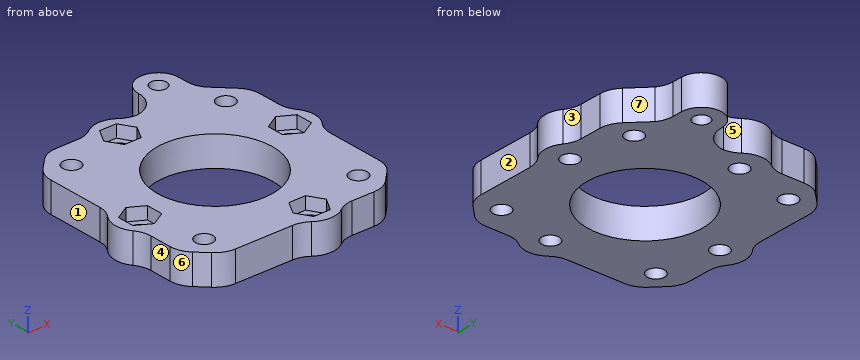
from build123d import *

# Parameters (mm, degrees)
SKETCH1_R           = 11.5
BOSS_EXTRUDE1_DEPTH = 6
SKETCH5_R           = 4.951700006
BOSS_EXTRUDE3_DEPTH = 6
SKETCH2_R           = 1.75
CUT_EXTRUDE1_DEPTH  = 34.075670817
SKETCH3_R           = 1.75
CUT_EXTRUDE2_DEPTH  = 34.075670817
CUT_EXTRUDE3_DEPTH  = 2.5
SKETCH6_R           = 1.6
BOSS_EXTRUDE4_DEPTH = 6
FILLET1_R           = 5


with BuildPart() as part:
    # Sketch1 → Boss-Extrude1 (new body)
    with BuildSketch(Plane.XY):
        Polygon((-21, 16), (-16, 21), (16, 21), (21, 16), (21, -16), (16, -21), (-16, -21), (-21, -16), align=None)
        Circle(SKETCH1_R, mode=Mode.SUBTRACT)
    extrude(amount=BOSS_EXTRUDE1_DEPTH)

    # Sketch5 → Boss-Extrude3 (add)
    with BuildSketch(Plane(origin=(0, 0, 0), x_dir=(-1, 0, 0), z_dir=(0, 0, -1))):
        with Locations((-18.048299994, 3.501266534)):
            Circle(SKETCH5_R)
        with Locations((3.501266534, 18.048299994)):
            Circle(SKETCH5_R)
        with Locations((18.048299994, -3.501266534)):
            Circle(SKETCH5_R)
        with Locations((-3.501266534, -18.048299994)):
            Circle(SKETCH5_R)
    extrude(amount=-BOSS_EXTRUDE3_DEPTH)

    # Sketch2 → Cut-Extrude1 (cut, through all)
    with BuildSketch(Plane.XY.offset(6)):
        with Locations((-15.5, 15.5)):
            Circle(SKETCH2_R)
        with Locations((15.5, 15.5)):
            Circle(SKETCH2_R)
        with Locations((15.5, -15.5)):
            Circle(SKETCH2_R)
        with Locations((-15.5, -15.5)):
            Circle(SKETCH2_R)
    extrude(amount=-CUT_EXTRUDE1_DEPTH, mode=Mode.SUBTRACT)

    # Sketch3 → Cut-Extrude2 (cut, through all)
    with BuildSketch(Plane.XY.offset(6)):
        with Locations((-3.501266534, 18.048299994)):
            Circle(SKETCH3_R)
        with Locations((18.048299994, 3.501266534)):
            Circle(SKETCH3_R)
        with Locations((3.501266534, -18.048299994)):
            Circle(SKETCH3_R)
        with Locations((-18.048299994, -3.501266534)):
            Circle(SKETCH3_R)
    extrude(amount=-CUT_EXTRUDE2_DEPTH, mode=Mode.SUBTRACT)

    # Sketch4 → Cut-Extrude3 (cut)
    with BuildSketch(Plane.XY.offset(6)):
        Polygon((-0.152634973, 18.048299994), (-1.826950753, 20.948299994), (-5.175582315, 20.948299994), (-6.849898095, 18.048299994), (-5.175582315, 15.148299994), (-1.826950753, 15.148299994), align=None)
        Polygon((18.048299994, 6.849898095), (15.148299994, 5.175582315), (15.148299994, 1.826950753), (18.048299994, 0.152634973), (20.948299994, 1.826950753), (20.948299994, 5.175582315), align=None)
        Polygon((-18.048299994, -6.849898095), (-15.148299994, -5.175582315), (-15.148299994, -1.826950753), (-18.048299994, -0.152634973), (-20.948299994, -1.826950753), (-20.948299994, -5.175582315), align=None)
        Polygon((6.849898095, -18.048299994), (5.175582315, -15.148299994), (1.826950753, -15.148299994), (0.152634973, -18.048299994), (1.826950753, -20.948299994), (5.175582315, -20.948299994), align=None)
    extrude(amount=-CUT_EXTRUDE3_DEPTH, mode=Mode.SUBTRACT)

    # Sketch6 → Boss-Extrude4 (add)
    with BuildSketch(Plane(origin=(0, 0, 0), x_dir=(-1, 0, 0), z_dir=(0, 0, -1))):
        with BuildLine():
            Line((-15, 26), (-15, 21))
            Line((-15, 21), (-7, 21))
            Line((-7, 21), (-7, 26))
            ThreePointArc((-7, 26), (-11, 30), (-15, 26))
        make_face()
        with Locations((-11, 26)):
            Circle(SKETCH6_R, mode=Mode.SUBTRACT)
    extrude(amount=-BOSS_EXTRUDE4_DEPTH)

    # Fillet1
    # the kernel refuses this fillet: 5 mm, written as the material it adds along each edge
    with BuildSketch(Plane(origin=(15, 21, 0), x_dir=(1, 0, 0), z_dir=(0, 0, 1))) as fillet1_piece_1:
        with BuildLine():
            CenterArc((5, 3), FILLET1_R, 180, 36.869897646)
            Line((0, 3), (0, 0))
            Line((0, 0), (1, 0))
        make_face()
    extrude(amount=6)
    with BuildSketch(Plane(origin=(7, 21, 0), x_dir=(-1, 0, 0), z_dir=(0, 0, 1))) as fillet1_piece_2:
        with BuildLine():
            CenterArc((FILLET1_R, -FILLET1_R), FILLET1_R, 90, 90)
            Line((0, -FILLET1_R), (0, 0))
            Line((0, 0), (FILLET1_R, 0))
        make_face()
    extrude(amount=6)
    with BuildSketch(Plane(origin=(7.477043191, -21, 6), x_dir=(-0.7048105163679362, -0.7093956131927819, 0), z_dir=(0, 0, -1)), Plane(origin=(-21, -7.477043191, 6), x_dir=(-0.7093956131927642, 0.7048105163679541, 0), z_dir=(0, 0, -1))) as fillet1_piece_3:
        with BuildLine():
            CenterArc((2.13164688, -4.948591109), FILLET1_R, 98.223270181, 36.962491831)
            Line((-1.415331186, -1.424538527), (0, 0))
            ThreePointArc((0, 0), (0.708246162, -0.050912281), (1.416492325, 0))
        make_face()
    extrude(amount=6)
    with BuildSketch(Plane(origin=(-0.474510123, -21, 6), x_dir=(-1, 0, 0), z_dir=(0, 0, -1)), Plane(origin=(-21, 0.474510123, 6), x_dir=(0, 1, 0), z_dir=(0, 0, -1))) as fillet1_piece_4:
        with BuildLine():
            CenterArc((2.008101686, -5), FILLET1_R, 90, 36.962491831)
            ThreePointArc((-0.998358687, -1.004853441), (-0.463062395, -0.538310232), (0, 0))
            Line((0, 0), (2.008101686, 0))
        make_face()
    extrude(amount=6)
    with BuildSketch(Plane(origin=(-7.477043191, 21, 6), x_dir=(-1, 0, 0), z_dir=(0, 0, -1)), Plane(origin=(21, 7.477043191, 6), x_dir=(0, 1, 0), z_dir=(0, 0, -1))) as fillet1_piece_5:
        with BuildLine():
            CenterArc((2.008101686, 5), FILLET1_R, 233.037508169, 36.962491831)
            ThreePointArc((-0.998358687, 1.004853441), (-0.463062395, 0.538310232), (0, 0))
            Line((0, 0), (2.008101686, 0))
        make_face()
    extrude(amount=6)
    with BuildSketch(Plane(origin=(0.474510123, 21, 6), x_dir=(-0.7048105163680716, 0.7093956131926475, 0), z_dir=(0, 0, -1)), Plane(origin=(21, -0.474510123, 6), x_dir=(0.7093956131926695, 0.7048105163680495, 0), z_dir=(0, 0, -1))) as fillet1_piece_6:
        with BuildLine():
            CenterArc((2.13164688, 4.948591109), FILLET1_R, 224.814237988, 36.962491831)
            Line((-1.415331186, 1.424538527), (0, 0))
            ThreePointArc((0, 0), (0.708246162, 0.050912281), (1.416492325, 0))
        make_face()
    extrude(amount=6)
    # the kernel refuses this fillet: 5 mm, written as the material it takes off along each edge
    with BuildSketch(Plane(origin=(21, -16, -5.17766953), x_dir=(0, 1, 0), z_dir=(0, 0, 1)), Plane(origin=(16, -21, -5.17766953), x_dir=(0.7071067811865476, 0.7071067811865476, 0), z_dir=(0, 0, 1)), Plane(origin=(-16, -21, -5.17766953), x_dir=(1, 0, 0), z_dir=(0, 0, 1)), Plane(origin=(-21, -16, -5.17766953), x_dir=(0.7071067811865476, -0.7071067811865476, 0), z_dir=(0, 0, 1)), Plane(origin=(-16, 21, -5.17766953), x_dir=(-0.7071067811865476, -0.7071067811865476, 0), z_dir=(0, 0, 1)), Plane(origin=(21, 16, -5.17766953), x_dir=(-0.7071067811865476, 0.7071067811865476, 0), z_dir=(0, 0, 1))) as fillet1_2_piece_1:
        with BuildLine():
            CenterArc((FILLET1_R * 0.414213562373, FILLET1_R), FILLET1_R, 225, 45)
            Line((-FILLET1_R * 0.292893218813, FILLET1_R * 0.292893218813), (0, 0))
            Line((0, 0), (FILLET1_R * 0.414213562373, 0))
        make_face()
    extrude(amount=16.355339059, mode=Mode.SUBTRACT)
    with BuildSketch(Plane(origin=(-21, 16, -5.17766953), x_dir=(0.7071067811865476, 0.7071067811865476, 0), z_dir=(0, 0, 1))) as fillet1_2_piece_2:
        with BuildLine():
            CenterArc((FILLET1_R * 0.414213562373, -FILLET1_R), FILLET1_R, 90, 45)
            Line((-FILLET1_R * 0.292893218813, -FILLET1_R * 0.292893218813), (0, 0))
            Line((0, 0), (FILLET1_R * 0.414213562373, 0))
        make_face()
    extrude(amount=16.355339059, mode=Mode.SUBTRACT)


solid = part.part
Input: part model. Units: mm. Frame: model coordinates. Face numbers are marked on the shaded views. A direction names the side the tool comes from. Round coordinates to 2 decimals unless told otherwise and drop trailing zeros. Write each loop counter-clockwise with the first axis right and the second up, starting at its lowest first coordinate (ties: lowest second). Pieces come first, ordered by that corner, then holes.
1) Contact query for flat-ended pins moving along their axis: P1, Ø1.3, axis at x = -11, z = 4.5, coming from the +Y side; P2, Ø2, axis at y = 24.5, z = 2.5, coming from the +X side; P3, Ø2, axis at y = 6.5, z = 3.5, coming from the +X side; P4, Ø3, axis at x = -3.5, y = 18.05, coming from the +Z side. Output: stop coordinate, or through.
2) Cut plane B-B (z = 2.75). Count the separate pieces of the cut face and the enclosed holes in it, then the cut area to 3 significant figures.
3) Reachability of the marked faces 1, 2, 3 and 4 from +Z, -Z, +X, -X, +Y, -Y: full face, straight path, thin tool, end or side. Return the list, or none.
4) Cut plane A-A (y = 27). Return the cut outline in (x, z).
5) Ray query, L1, parallel to X at y = -5, z = 0.75; L2, parallel to Y at x = -17, z = 3.25; L3, parallel to Y at x = -4.5, z = 1. Return the intervals inside material, ascending.
6) Draft query along X for the marked faces 5, 6 and 7. Return one class per face: pulls with the +X half, pulls with the -X half, needs draft (parallel to the pull), parting line crosses it, or undercut.
Geometry says:
1. P1: stops at y = 21
1. P2: stops at x = 15.03
1. P3: stops at x = 22.58
1. P4: passes through
2. separate pieces: 1
2. enclosed holes: 10
2. area: 1,330 mm2
3. face 1: +Z, -Z, -X, +Y
3. face 2: +Z, -Z, +X, -Y
3. face 3: +Z, -Z, +X, +Y
3. face 4: +Z, -Z, -X, -Y
4. outline: (7.13, 0) - (9.75, 0) - (9.75, 6) - (7.13, 6) - close; (12.25, 0) - (14.87, 0) - (14.87, 6) - (12.25, 6) - close
5. L1: x = -22.77 to -18.95, -17.14 to -10.36, 10.36 to 21
5. L2: y = -19.95 to -16.4, -14.6 to -4.9, -2.1 to 14.6, 16.4 to 19.95
5. L3: y = -21 to -10.58, 10.58 to 16.61, 19.49 to 22.9
6. face 5: undercut
6. face 6: pulls with the -X half
6. face 7: pulls with the +X half
